Design review of the part built by this model. Coordinates are the model's own, in mm. A direction names the side the tool comes from. Coordinates: 2 decimals unless noted, no trailing zeros. Loops run counter-clockwise (first coordinate to the right, second up) from the corner with the lowest first, then second, coordinate; pieces in that order, holes last.
Q1. Add section B-B on z = 3.75. Give the boundary of the cut face in (x, y).
Q2. Machinability: for faces 1 (the face through (45, 28, 19)), 2 (the face through (-4, 28, 1)), 3 (the face through (45, 29.4, 10)), 4 (the face through (35.39, 36.46, 7.51)), 5 (the face through (45, 28, 1)), which of the approach directions +Z, -Z, +X, -X, +Y, -Y give a long, thin tool a straight path to every point of the face, cutting with its end or side? Answer none if there is none.
Q3. Draft analysis for pull direction Y (two halves, no side actions). For faces 6 (the face through (20, 0, 10)), 7 (the face through (48.5, 28, 10)), 8 (the face through (35, 39.5, 6)), state which applies: released by +Y, released by -Y, zero draft, split by the parting line, or undercut.
Q4. Add section A-A on x = 21. Give the boundary of the cut face in (y, z).
Q5. For P1, Ø8, axis at x = 45.5, z = 8, coming from the -Y side; P2, Ø10.5, axis at x = 31, z = 12.5, coming from the -Y side; P3, Ø1.5, axis at x = 30.5, y = 12, coming from the -Z side; P4, Ø2.5, axis at x = -2, y = 28.5, coming from the +Z side, all flat-tipped, find the tip position at first contact; note any pin that passes through.
Q6. Add section D-D on z = 10. Give the boundary of the cut face in (x, y), and give its area (3 significant figures).
Q7. Wall thickness on probe 1 along Y at (x, z) = (22.5, 11.5); probe 2 along X at (y, z) = (9, 6.25); probe 3 along Z at (x, y) = (11.5, 29.5): over which ranges is each line inside the solid? List them lowest first.
Q8. Add section C-C on x = 30.6. Give the boundary of the cut face in (y, z), and give its area (3 significant figures).
```python
from build123d import *

# Parameters (mm, degrees)
SKETCH1_W           = 41
SKETCH1_H           = 33.5
BOSS_EXTRUDE1_DEPTH = 20
SKETCH3_W           = 18
SKETCH3_H           = 2.4
BOSS_EXTRUDE2_DEPTH = 7.5


with BuildPart() as part:
    # Sketch1 → Boss-Extrude1 (new body)
    with BuildSketch(Plane.XY):
        with Locations((20.5, 16.75)):
            Rectangle(SKETCH1_W, SKETCH1_H)
    extrude(amount=BOSS_EXTRUDE1_DEPTH)

    # Sketch3 → Boss-Extrude2 (add)
    with BuildSketch(Plane(origin=(41, 0, 0), x_dir=(0, 0, -1), z_dir=(1, 0, 0))):
        with Locations((-10, 28.2)):
            Rectangle(SKETCH3_W, SKETCH3_H)
    boss_extrude2 = extrude(amount=BOSS_EXTRUDE2_DEPTH)

    # Mirror1: Boss-Extrude2 across plane
    add(boss_extrude2.mirror(Plane(origin=(20.5, 0, 0), x_dir=(0, 0, 1), z_dir=(1, 0, 0))))

    # Sketch5 → Revolve1 (revolve)
    with BuildSketch(Plane.XY.offset(10), mode=Mode.PRIVATE) as revolve1_sk:
        Polygon((30.6, 33.5), (30.6, 41.5), (41, 41.5), (41, 39.5), (36, 39.5), (36, 33.5), align=None)
    revolve(revolve1_sk.sketch.rotate(Axis((30.6, 33.5, 10), (0, 1, 0)), 90), axis=Axis((30.6, 33.5, 10), (0, 1, 0)))


solid = part.part
```
Entries:
1. outline: (-7.5, 27) - (0, 27) - (0, 0) - (41, 0) - (41, 27) - (48.5, 27) - (48.5, 29.4) - (41, 29.4) - (41, 33.5) - (0, 33.5) - (0, 29.4) - (-7.5, 29.4) - close; (22.29, 39.5) - (38.91, 39.5) - (38.91, 41.5) - (22.29, 41.5) - close
2. face 1: +Z, +X, +Y, -Y
2. face 2: -Z, -X, +Y, -Y
2. face 3: +Z, -Z, +X, +Y
2. face 4: none
2. face 5: -Z, +X, +Y, -Y
3. face 6: released by -Y
3. face 7: zero draft
3. face 8: undercut
4. outline: (0, 0) - (33.5, 0) - (33.5, 20) - (0, 20) - close; (39.5, 6) - (41.5, 6) - (41.5, 14) - (39.5, 14) - close
5. P1: stops at y = 27
5. P2: stops at y = 0
5. P3: stops at z = 0
5. P4: stops at z = 19
6. outline: (-7.5, 27) - (0, 27) - (0, 0) - (41, 0) - (41, 27) - (48.5, 27) - (48.5, 29.4) - (41, 29.4) - (41, 33.5) - (36, 33.5) - (36, 39.5) - (41, 39.5) - (41, 41.5) - (20.2, 41.5) - (20.2, 39.5) - (25.2, 39.5) - (25.2, 33.5) - (0, 33.5) - (0, 29.4) - (-7.5, 29.4) - close
6. area: 1,520 mm2
7. probe 1: y = 0 to 33.5, 39.5 to 41.5
7. probe 2: x = 0 to 41
7. probe 3: z = 0 to 20
8. outline: (0, 0) - (33.5, 0) - (33.5, 4.6) - (39.5, 4.6) - (39.5, -0.4) - (41.5, -0.4) - (41.5, 20.4) - (39.5, 20.4) - (39.5, 15.4) - (33.5, 15.4) - (33.5, 20) - (0, 20) - close
8. area: 776 mm2
